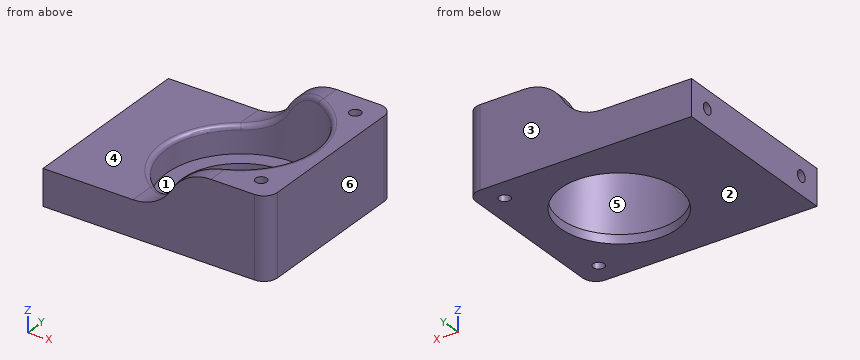
```python
from build123d import *

# Parameters (mm, degrees)
SKETCH_1_W          = 50
SKETCH_1_H          = 40
EXTRUDE_1_DEPTH     = 8
SKETCH_2_W          = 20
SKETCH_2_H          = 40
EXTRUDE_2_DEPTH     = 10
SKETCH_3_R          = 16.5
CUT_EXTRUDE_1_DEPTH = 16
SKETCH_5_R          = 1.25
CUT_EXTRUDE_2_DEPTH = 37.728735344
SKETCH_6_R          = 1.25
CUT_EXTRUDE_3_DEPTH = 10
FILLET_1_R          = 10
FILLET_2_R          = 10
FILLET_3_R          = 3
SKETCH_7_R          = 13
CUT_EXTRUDE_4_DEPTH = 36.791060507
FILLET_4_R          = 1


with BuildPart() as part:
    # 草图1 → 凸台-拉伸1 (new body)
    with BuildSketch(Plane.XY):
        Rectangle(SKETCH_1_W, SKETCH_1_H)
    extrude(amount=EXTRUDE_1_DEPTH)

    # 草图2 → 凸台-拉伸2 (add)
    with BuildSketch(Plane.XY.offset(8)):
        with Locations((15, 0)):
            Rectangle(SKETCH_2_W, SKETCH_2_H)
    extrude(amount=EXTRUDE_2_DEPTH)

    # 草图3 → 切除-拉伸1 (cut)
    with BuildSketch(Plane.XY.offset(18)):
        with Locations((5, 0)):
            Circle(SKETCH_3_R)
    extrude(amount=-CUT_EXTRUDE_1_DEPTH, mode=Mode.SUBTRACT)

    # 草图5 → 切除-拉伸2 (cut, through all)
    with BuildSketch(Plane.XY.offset(18)):
        with Locations((20, 15)):
            Circle(SKETCH_5_R)
        with Locations(Location((20, -15, 0), (0, 0, 180))):
            Circle(SKETCH_5_R)
    extrude(amount=-CUT_EXTRUDE_2_DEPTH, mode=Mode.SUBTRACT)

    # 草图6 → 切除-拉伸3 (cut)
    with BuildSketch(Plane.ZY.offset(25)):
        with Locations((4, 15)):
            Circle(SKETCH_6_R)
        with Locations(Location((4, -15, 0), (0, 0, 180))):
            Circle(SKETCH_6_R)
    extrude(amount=-CUT_EXTRUDE_3_DEPTH, mode=Mode.SUBTRACT)

    # 圆角1
    fillet_1_edges = [part.edges().sort_by_distance(p)[0] for p in [
        (5, -18.25, 8),
        (5, 18.25, 8),
    ]]
    fillet(fillet_1_edges, radius=FILLET_1_R - 0.0001)  # a hair under: the kernel refuses the full size

    # 圆角2
    fillet_2_edges = [part.edges().sort_by_distance(p)[0] for p in [
        (5, -18.25, 18),
        (5, 18.25, 18),
    ]]
    fillet(fillet_2_edges, radius=FILLET_2_R)

    # 圆角3
    fillet_3_edges = [part.edges().sort_by_distance(p)[0] for p in [
        (25, -20, 9),
        (25, 20, 9),
    ]]
    fillet(fillet_3_edges, radius=FILLET_3_R)

    # 草图7 → 切除-拉伸4 (cut, through all)
    with BuildSketch(Plane.XY.offset(2)):
        with Locations((5, 0)):
            Circle(SKETCH_7_R)
    extrude(amount=-CUT_EXTRUDE_4_DEPTH, mode=Mode.SUBTRACT)

    # 圆角4
    fillet_4_edges = [part.edges().sort_by_distance(p)[0] for p in [
        (-11.5, 0, 8),
        (-0.245631372, -15.643955751, 9.202461182),
        (19.018542731, -8.702324959, 18),
        (-0.245631372, 15.643955751, 9.202461182),
        (7.42567519, 16.320726083, 16.720103053),
        (7.42567519, -16.320726083, 16.720103053),
    ]]
    fillet(fillet_4_edges, radius=FILLET_4_R)


solid = part.part
```
CAD build for the part. Positions are in the model's coordinates, mm. Face numbers are marked on the shaded views. A direction names the side the tool comes from. Round coordinates to 2 decimals unless told otherwise and drop trailing zeros. Order: outer loops, then holes, each group sorted by start corner. A loop starts at its lowest first (then second) coordinate and runs counter-clockwise, first axis right, second up.
Q1. Wall check: L1, parallel to X at y = 0, z = 4; L2, parallel to Y at x = 5, z = 0.7; L3, parallel to Z at x = -18.5, y = -15. Give the ranges that are in metal, low to high.
Q2. Which spindle directions (+Z, -Z, +X, -X, +Y, -Y) get a long thin tool onto all of the face, cutting with end or side? Do the marked faces 4, 5 and 6. Say none if no direction does.
Q3. Two-plate mould, pull along Z, no slides. Class the marked faces 1, 2 and 3: pulls with the +Z half, pulls with the -Z half, needs draft (parallel to the pull), parting line crosses it, or undercut.
Q4. Slice it at B-B (y = 0). Write the cut outline in (x, z).
Q5. Slice it at A-A (z = 6). Write the cut outline in (x, y).
Q6. Drop flat-ended pins along their axis: pin 1 (12 mm diameter, centred on x = -11, y = 15.5, fed in from +Z); pin 2 (23.5 mm diameter, centred on x = 5, y = 0, fed in from -Z). Give the stop position or say it passes through.
Q7. Slice it at C-C (x = 20). State how many separate pieces and enclosed holes the cut face has, and give its area (3 significant figures).
Results below:
1. L1: x = -25 to -11.5, 21.5 to 25
1. L2: y = -20 to -13, 13 to 20
1. L3: z = 0 to 2.75, 5.25 to 8
2. face 4: +Z, -X, +Y, -Y
2. face 5: +Z
2. face 6: +Z, -Z, +X, +Y, -Y
3. face 1: pulls with the +Z half
3. face 2: pulls with the -Z half
3. face 3: needs draft
4. outline: (-25, 0) - (-8, 0) - (-8, 2) - (-11.5, 2) - (-11.5, 7) arc R1 ccw to (-12.5, 8) - (-25, 8) - close; (18, 0) - (25, 0) - (25, 18) - (22.5, 18) arc R1 ccw to (21.5, 17) - (21.5, 2) - (18, 2) - close
5. outline: (-25, -20) - (22, -20) arc R3 ccw to (25, -17) - (25, 17) arc R3 ccw to (22, 20) - (-25, 20) - close; hole circle Ø33 at (5, 0); hole circle Ø2.5 at (20, -15); hole circle Ø2.5 at (20, 15)
6. pin 1: stops at z = 8
6. pin 2: passes through
7. separate pieces: 3
7. enclosed holes: 0
7. area: 409 mm2
